Here's how the part is built. I have some questions about the finished solid (model axes, mm). A direction names the side the tool comes from. Coordinates: 2 decimals unless noted, no trailing zeros. Write each loop counter-clockwise with the first axis right and the second up, starting at its lowest first coordinate (ties: lowest second). Pieces come first, ordered by that corner, then holes.
(1) Imagine slicing it at C-C, the plane x = 2.5. List the corners of the cut face in (y, z) for me.
(2) Imagine slicing it at B-B, the plane y = -39. List the corners of the cut face in (x, z) for me, plus the area to 3 significant figures.
(3) Imagine slicing it at A-A, the plane z = -10. List the corners of the cut face in (x, y) for me.
(4) Imagine slicing it at D-D, the plane z = -39. List the corners of the cut face in (x, y) for me, plus the area to 3 significant figures.
(5) Thinking about a two-plate mould opening in Z: for faces 1 (the flat face through (0, -1, -1)), 2 (the cylindrical face through (0.07, -17.81, -8.27)), 3 (the flat face through (0, -14, -44)), which applies, released by +Z, released by -Z, zero draft, split by the parting line, or undercut?
(6) Please list where these lines run through material, in increasing order: probe 1 along Y at (x, z) = (-2.5, -10); probe 2 along Z at (x, y) = (-1.25, -8); probe 3 along Y at (x, z) = (-3.5, -34.5).
(7) For pin 1 Ø6 at (x, y) = (1.5, -42) entering from -Z; pin 2 Ø10 at (y, z) = (-16.5, -7.5) entering from +X; pin 3 Ø9.5 at (y, z) = (-10, -10) entering from +X; pin 4 Ø3 at (x, z) = (-0.5, -36) entering from -Y, each with a flat end and sliding along its axis, tell me the tip position at first contact or that it passes through.
(8) Which directions (+Z, -Z, +X, -X, +Y, -Y) give clear straight access to the entire face, cutting with the end or side of a thin tool? Please do faces 4 (the flat face through (0, -48, -1)), 5 (the flat face through (0, -36, -20)).
```python
from build123d import *

# Parameters (mm, degrees)
SKETCH1_W              = 45
SKETCH1_H              = 49
BOSS_EXTRUDE1_DEPTH    = 5
SKETCH2_W              = 25
SKETCH2_H              = 34
CUT_EXTRUDE1_DEPTH     = 68.275552766
SKETCH3_R              = 8
CUT_EXTRUDE2_DEPTH     = 68.275552766
M8X1_25_TAPPED_HOLE1_D = 6.8
M6X1_0_TAPPED_HOLE1_D  = 5
FILLET1_R              = 10
CHAMFER1_SIZE          = 2


with BuildPart() as part:
    # Sketch1 → Boss-Extrude1 (new, symmetric)
    with BuildSketch(Plane(origin=(0, 0, 0), x_dir=(0, 0, -1), z_dir=(1, 0, 0))):
        with Locations((22.5, -24.5)):
            Rectangle(SKETCH1_W, SKETCH1_H)
    extrude(amount=BOSS_EXTRUDE1_DEPTH, both=True)

    # Sketch2 → Cut-Extrude1 (cut, through all)
    with BuildSketch(Plane(origin=(5, 0, 0), x_dir=(0, 0, -1), z_dir=(1, 0, 0))):
        with Locations((32.5, -32)):
            Rectangle(SKETCH2_W, SKETCH2_H)
    extrude(amount=-CUT_EXTRUDE1_DEPTH, mode=Mode.SUBTRACT)

    # Sketch3 → Cut-Extrude2 (cut, through all)
    with BuildSketch(Plane(origin=(5, 0, 0), x_dir=(0, 0, -1), z_dir=(1, 0, 0))):
        with Locations((10, -10)):
            Circle(SKETCH3_R)
    extrude(amount=-CUT_EXTRUDE2_DEPTH, mode=Mode.SUBTRACT)

    # M8x1.25 Tapped Hole1 (through all)
    with Locations(Plane(origin=(5, 0, 0), x_dir=(0, 0, -1), z_dir=(1, 0, 0))):
        with Locations((10, -39)):
            Hole(M8X1_25_TAPPED_HOLE1_D / 2)

    # M6x1.0 Tapped Hole1 (through all)
    with Locations(Plane(origin=(5, 0, 0), x_dir=(0, 0, -1), z_dir=(1, 0, 0))):
        with Locations((39, -7)):
            Hole(M6X1_0_TAPPED_HOLE1_D / 2)

    # Fillet1
    fillet1_edges = [part.edges().sort_by_distance(p)[0] for p in [
        (0, -15, -20),
    ]]
    fillet(fillet1_edges, radius=FILLET1_R)

    # Chamfer1
    chamfer1_edges = [part.edges().sort_by_distance(p)[0] for p in [
        (0, -15, -45),
        (0, -49, -20),
        (0, 0, 0),
        (0, 0, -45),
        (0, -49, 0),
    ]]
    chamfer(chamfer1_edges, length=CHAMFER1_SIZE)


solid = part.part
```
Recorded:
1. outline: (-49, -18) - (-47, -20) - (-25, -20) arc R10 cw to (-15, -30) - (-15, -43) - (-13, -45) - (-2, -45) - (0, -43) - (0, -2) - (-2, 0) - (-47, 0) - (-49, -2) - close; hole circle Ø6.8 at (-39, -10); hole circle Ø16 at (-10, -10); hole circle Ø5 at (-7, -39)
2. outline: (-5, -20) - (5, -20) - (5, -13.4) - (-5, -13.4) - close; (-5, -6.6) - (5, -6.6) - (5, 0) - (-5, 0) - close
2. area: 132 mm2
3. outline: (-5, -49) - (5, -49) - (5, -42.4) - (-5, -42.4) - close; (-5, -35.6) - (5, -35.6) - (5, -18) - (-5, -18) - close; (-5, -2) - (5, -2) - (5, 0) - (-5, 0) - close
4. outline: (-5, -15) - (5, -15) - (5, -9.5) - (-5, -9.5) - close; (-5, -4.5) - (5, -4.5) - (5, 0) - (-5, 0) - close
4. area: 100 mm2
5. face 1: released by +Z
5. face 2: undercut
5. face 3: released by -Z
6. probe 1: y = -49 to -42.4, -35.6 to -18, -2 to 0
6. probe 2: z = -45 to -41.29, -36.71 to -17.75, -2.25 to 0
6. probe 3: y = -15 to 0
7. pin 1: stops at z = -20
7. pin 2: stops at x = 5
7. pin 3: passes through
7. pin 4: stops at y = -15
8. face 4: +Z, +X, -X, -Y
8. face 5: -Z, +X, -X, -Y
